Work out the finished part from the listing and answer in its coordinate system (mm). A direction names the side the tool comes from. Coordinates: 2 decimals unless noted, no trailing zeros. Order: outer loops, then holes, each group sorted by start corner. A loop starts at its lowest first (then second) coordinate and runs counter-clockwise, first axis right, second up. Notation, with made-up numbers: (-2, -10.5) -> (18, -10.5) arc R18 cw to (18, 22.5) -> close; hole circle Ø2 at (-17, 10.5). An arc over 180 degrees is marked (long way). Write item = value, one per line. Start each with the question number.
Q1. Which of the six approach directions +Z, -Z, +X, -X, +Y, -Y give full straight-line access (tool end or side, diameter ignored) to faces 1 (the cylindrical face through (71.369, 12.93, 1.915)), 2 (the cylindrical face through (70.32, 3.94, -19.5)), 3 (the flat face through (-15, 4, 18))?
Q2. Flat-ended cylindrical pins translate along their axes: pin 1 (6.5 mm diameter, centred on x = 22.5, z = 16, fed in from +Y); pin 2 (1 mm diameter, centred on x = 42, z = -8, fed in from +Y). Find the tip coordinate at first contact, or state that the pin passes through.
Q3. For a pull along Z with two mould halves and no side action, classify faces 4 (the flat face through (2, 5, 21)), 5 (the flat face through (-53, 8, 0)), 6 (the cylindrical face through (58.419, 0.986, 17.526)) as +Z half, -Z half, draft (parallel to the pull), parting line (faces both ways), or undercut.
Q4. The part is cut by section D-D, the plane x = -18. Determine the outline of the cut face in (y, z).
Q5. The part is cut by section B-B, the plane x = 39.75. Determine the outline of the cut face in (y, z), plus the area to 3 significant figures.
Q6. The part is cut by section C-C, the plane x = 22.75. Determine the outline of the cut face in (y, z).
Q7. Straight lines are drawn through the part: L1, parallel to X at y = 6.5, z = -19; L2, parallel to X at y = 1.5, z = -6; L3, parallel to Z at x = 66.75, y = 8.5. For each, find the intervals that lie inside material, in ascending order. Write a range as from..to.
Q8. The part is cut by section A-A, the plane y = 10.5. Determine the outline of the cut face in (x, z), plus the area to 3 significant figures.
```python
from build123d import *

# Parameters (mm, degrees)
SKETCH1_W           = 123.5
SKETCH1_H           = 42
BOSS_EXTRUDE1_DEPTH = 8
SKETCH2_R           = 11.2
CUT_EXTRUDE1_DEPTH  = 7
CUT_EXTRUDE2_REACH  = 10
SKETCH3_R           = 7.55
CUT_EXTRUDE4_DEPTH  = 6
SKETCH10_R          = 1.75
CUT_EXTRUDE5_DEPTH  = 2
SKETCH12_W          = 6
SKETCH12_H          = 10
BOSS_EXTRUDE2_DEPTH = 42
SKETCH13_W          = 57
SKETCH13_H          = 36
CUT_EXTRUDE6_DEPTH  = 9
SKETCH23_W          = 10
SKETCH23_H          = 42
BOSS_EXTRUDE3_DEPTH = 8
SKETCH24_R          = 5
BOSS_EXTRUDE4_DEPTH = 10
FILLET1_R           = 5
SKETCH25_R          = 2.35
CUT_EXTRUDE7_DEPTH  = 18


with BuildPart() as part:
    # Sketch1 → Boss-Extrude1 (new body)
    with BuildSketch(Plane(origin=(0, 0, 0), x_dir=(1, 0, 0), z_dir=(0, 1, 0))):
        Rectangle(SKETCH1_W, SKETCH1_H)
    extrude(amount=BOSS_EXTRUDE1_DEPTH)

    # Sketch2 → Cut-Extrude1 (cut)
    with BuildSketch(Plane(origin=(0, 8, 0), x_dir=(1, 0, 0), z_dir=(0, 1, 0))):
        with Locations((39.75, 0)):
            Circle(SKETCH2_R)
    extrude(amount=-CUT_EXTRUDE1_DEPTH, mode=Mode.SUBTRACT)

    # Sketch3 → Cut-Extrude2 (cut, up to next)
    with BuildSketch(Plane.XZ, mode=Mode.PRIVATE) as cut_extrude2_sk1:
        with Locations((39.75, 0)):
            Circle(SKETCH3_R)
    cut_extrude2_tool1 = extrude(cut_extrude2_sk1.sketch, amount=-CUT_EXTRUDE2_REACH, mode=Mode.PRIVATE) & part.part
    add(cut_extrude2_tool1.solids().sort_by_distance((39.75, 0, 0))[0], mode=Mode.SUBTRACT)

    # Sketch9 → Cut-Extrude4 (cut)
    with BuildSketch(Plane(origin=(0, 8, 0), x_dir=(1, 0, 0), z_dir=(0, 1, 0))):
        Polygon((58.482050808, 20), (55.017949192, 20), (53.285898385, 17), (55.017949192, 14), (58.482050808, 14), (60.214101615, 17), align=None)
        Polygon((60.214101615, -17), (58.482050808, -20), (55.017949192, -20), (53.285898385, -17), (55.017949192, -14), (58.482050808, -14), align=None)
        Polygon((19.285898385, 17), (21.017949192, 20), (24.482050808, 20), (26.214101615, 17), (24.482050808, 14), (21.017949192, 14), align=None)
        Polygon((21.017949192, -14), (19.285898385, -17), (21.017949192, -20), (24.482050808, -20), (26.214101615, -17), (24.482050808, -14), align=None)
    extrude(amount=-CUT_EXTRUDE4_DEPTH, mode=Mode.SUBTRACT)

    # Sketch10 → Cut-Extrude5 (cut)
    with BuildSketch(Plane.XZ):
        with Locations((56.75, 17)):
            Circle(SKETCH10_R)
        with Locations((22.75, 17)):
            Circle(SKETCH10_R)
        with Locations((56.75, -17)):
            Circle(SKETCH10_R)
        with Locations((22.75, -17)):
            Circle(SKETCH10_R)
    extrude(amount=-CUT_EXTRUDE5_DEPTH, mode=Mode.SUBTRACT)

    # Sketch12 → Boss-Extrude2 (add)
    with BuildSketch(Plane(origin=(0, 0, -21), x_dir=(-1, 0, 0), z_dir=(0, 0, -1))):
        with Locations((58.75, 13)):
            Rectangle(SKETCH12_W, SKETCH12_H)
        Polygon((50.75, 8), (45.75, 8), (45.75, 13), align=None)
    extrude(amount=-BOSS_EXTRUDE2_DEPTH)

    # Sketch13 → Cut-Extrude6 (cut, through all)
    with BuildSketch(Plane(origin=(0, 8, 0), x_dir=(1, 0, 0), z_dir=(0, 1, 0))):
        with Locations((-14.25, 0)):
            Rectangle(SKETCH13_W, SKETCH13_H)
    extrude(amount=-CUT_EXTRUDE6_DEPTH, mode=Mode.SUBTRACT)

    # Sketch23 → Boss-Extrude3 (add)
    with BuildSketch(Plane(origin=(0, 8, 0), x_dir=(1, 0, 0), z_dir=(0, 1, 0))):
        with Locations((66.75, 0)):
            Rectangle(SKETCH23_W, SKETCH23_H)
    extrude(amount=-BOSS_EXTRUDE3_DEPTH)

    # Sketch24 → Boss-Extrude4 (add)
    with BuildSketch(Plane(origin=(0, 8, 0), x_dir=(1, 0, 0), z_dir=(0, 1, 0))):
        with Locations((66.75, 0)):
            Circle(SKETCH24_R)
    extrude(amount=BOSS_EXTRUDE4_DEPTH)

    # Fillet1
    fillet1_edges = [part.edges().sort_by_distance(p)[0] for p in [
        (71.75, 4, -21),
        (71.75, 4, 21),
    ]]
    fillet(fillet1_edges, radius=FILLET1_R)

    # Sketch25 → Cut-Extrude7 (cut)
    with BuildSketch(Plane(origin=(0, 18, 0), x_dir=(1, 0, 0), z_dir=(0, 1, 0))):
        with Locations((66.75, 0)):
            Circle(SKETCH25_R)
    extrude(amount=-CUT_EXTRUDE7_DEPTH, mode=Mode.SUBTRACT)


solid = part.part
```
Model answer:
q1.face_1 = +Y
q1.face_2 = -Z, +X, +Y, -Y
q1.face_3 = +Y, -Y
q2.pin_1 = 8
q2.pin_2 = 1
q3.face_4 = +Z half
q3.face_5 = draft
q3.face_6 = undercut
q4.outline = (0, -21) -> (8, -21) -> (8, -18) -> (0, -18) -> close; (0, 18) -> (8, 18) -> (8, 21) -> (0, 21) -> close
q5.outline = (0, -21) -> (8, -21) -> (8, -11.2) -> (1, -11.2) -> (1, -7.55) -> (0, -7.55) -> close; (0, 7.55) -> (1, 7.55) -> (1, 11.2) -> (8, 11.2) -> (8, 21) -> (0, 21) -> close
q5.area = 164 mm2
q6.outline = (0, -21) -> (8, -21) -> (8, -20) -> (2, -20) -> (2, -18.75) -> (0, -18.75) -> close; (0, -15.25) -> (2, -15.25) -> (2, -14) -> (8, -14) -> (8, 14) -> (2, 14) -> (2, 15.25) -> (0, 15.25) -> close; (0, 18.75) -> (2, 18.75) -> (2, 20) -> (8, 20) -> (8, 21) -> (0, 21) -> close
q7.L1 = -61.75..20.44, 25.06..54.44, 59.06..70.75
q7.L2 = -61.75..-42.75, 14.25..30.29, 49.21..71.75
q7.L3 = -5..-2.35, 2.35..5
q8.outline = (-61.75, -21) -> (-55.75, -21) -> (-55.75, 21) -> (-61.75, 21) -> close; (-48.25, -21) -> (-45.75, -21) -> (-45.75, 21) -> (-48.25, 21) -> close; circle Ø10 at (66.75, 0); hole circle Ø4.7 at (66.75, 0)
q8.area = 418 mm2
